```python
from build123d import *

# Parameters (mm, degrees)
BOSS_EXTRUDE1_DEPTH = 18
SKETCH3_R           = 1.5
CUT_EXTRUDE1_DEPTH  = 25.939927827
CHAMFER1_SIZE       = 2
BOSS_EXTRUDE2_DEPTH = 0.5
LPATTERN1_COUNT     = 8
LPATTERN1_PITCH     = 2
SKETCH5_W           = 0.5
SKETCH5_H           = 4.5
BOSS_EXTRUDE3_DEPTH = 0.5
LPATTERN2_COUNT     = 8
LPATTERN2_PITCH     = 2


with BuildPart() as part:
    # Sketch2 → Boss-Extrude1 (new body)
    with BuildSketch(Plane(origin=(0, 0, 0), x_dir=(0, 0, -1), z_dir=(1, 0, 0))):
        Polygon((0, 0), (0, 17), (-2, 17), (-2, 11), (-5, 11), (-5, 0), align=None)
    extrude(amount=BOSS_EXTRUDE1_DEPTH)

    # Sketch3 → Cut-Extrude1 (cut, through all)
    with BuildSketch(Plane.XY.offset(2)):
        with Locations((9, 14)):
            Circle(SKETCH3_R)
    extrude(amount=-CUT_EXTRUDE1_DEPTH, mode=Mode.SUBTRACT)

    # Chamfer1
    chamfer1_edges = [part.edges().sort_by_distance(p)[0] for p in [
        (18, 17, 1),
        (0, 17, 1),
    ]]
    chamfer(chamfer1_edges, length=CHAMFER1_SIZE)

    # Sketch4 → Boss-Extrude2 (add)
    with BuildSketch(Plane(origin=(2.227, 0, 0), x_dir=(0, 0, -1), z_dir=(1, 0, 0))):
        Polygon((-2.25, 0), (-2.25, -1), (-9.25, -1), (-9.25, -4.5), (-9.75, -4.5), (-9.75, -0.5), (-2.75, -0.5), (-2.75, 0), align=None)
    boss_extrude2 = extrude(amount=BOSS_EXTRUDE2_DEPTH)

    # LPattern1: Boss-Extrude2 ×8
    with Locations(*[(i * LPATTERN1_PITCH, 0, 0) for i in range(1, LPATTERN1_COUNT)]):
        add(boss_extrude2)

    # Sketch5 → Boss-Extrude3 (add)
    with BuildSketch(Plane(origin=(1.227, 0, 0), x_dir=(0, 0, -1), z_dir=(1, 0, 0))):
        with Locations((-2.5, -2.25)):
            Rectangle(SKETCH5_W, SKETCH5_H)
    boss_extrude3 = extrude(amount=BOSS_EXTRUDE3_DEPTH)

    # LPattern2: Boss-Extrude3 ×8
    with Locations(*[(i * LPATTERN2_PITCH, 0, 0) for i in range(1, LPATTERN2_COUNT)]):
        add(boss_extrude3)


solid = part.part
```
Work out the finished part from the listing and answer in its coordinate system (mm). A direction names the side the tool comes from. Give positions to 0.01 mm unless a question says otherwise; leave off trailing zeros. Loops run counter-clockwise (first coordinate to the right, second up) from the corner with the lowest first, then second, coordinate; pieces in that order, holes last. Notation, with made-up numbers: (-23.75, 70.25) -> (33.25, 70.25) arc R24 ccw to (33.25, 102.25) -> close; hole circle Ø6 at (-24, 69). An arc over 180 degrees is marked (long way). Put each result on its own line as item: value. Start each with the question number.
Item 1: The part is cut by section D-D (y = 8.5). Give the vertices of the cut face in (x, z), then the cut area to 3 significant figures.
Item 2: Which of the six approach directions +Z, -Z, +X, -X, +Y, -Y give full straight-line access (tool end or side, diameter ignored) to faces 5 (the face through (9, 11, 3)), 6 (the face through (0, 8, 3)), 7 (the face through (8.727, -0.7, 7.1))?
Item 3: The part is cut by section B-B (z = 8). State how many separate pieces and enclosed holes the cut face has, then the cut area to 3 significant figures.
Item 4: Each of these flat-tipped pins is pushed along its axis until it touches: P1, Ø0.6, axis at x = 11.5, y = -1.5, coming from the +Z side; P2, Ø6, axis at x = 3.5, y = 8, coming from the +Z side; P3, Ø1, axis at x = 14.5, z = 3.5, coming from the +Y side. Where does it stop, or does it pass through?
Item 5: Find the intervals of material crossed by L1, parallel to Y at x = 9, z = 0.8; L2, parallel to Z at x = 2.25, y = 5.5; L3, parallel to Y at x = 12.25, z = 0.5, in increasing order. Write a range as [from, to].
Item 6: The part is cut by section A-A (y = 14). Give the vertices of the cut face in (x, z).
Item 7: The mould has two halves that part along X. Classify faces 1 (the face through (18, 8, 3)), 2 (the face through (10.727, -0.7, 7.1)), 3 (the face through (9, 6, 5)), 4 (the face through (6.727, -0.7, 7.1)): released by +X, released by -X, zero draft, split by the parting line, or undercut.
Answers below:
1. outline: (0, 0) -> (18, 0) -> (18, 5) -> (0, 5) -> close
1. area: 90.0 mm2
2. face 5: +Z, +X, -X, +Y
2. face 6: +Z, -Z, -X, +Y, -Y
2. face 7: +Z, -Z, -Y
3. separate pieces: 8
3. enclosed holes: 0
3. area: 2.00 mm2
4. P1: z = 2.75
4. P2: z = 5
4. P3: y = 11
5. L1: [0, 12.5], [15.5, 17]
5. L2: [0, 5]
5. L3: [0, 17]
6. outline: (0, 0) -> (7.5, 0) -> (7.5, 2) -> (0, 2) -> close; (10.5, 0) -> (18, 0) -> (18, 2) -> (10.5, 2) -> close
7. face 1: released by +X
7. face 2: undercut
7. face 3: zero draft
7. face 4: undercut
